Check sheet for the modelled part. Datum: model origin and axes. Units: mm. Face numbers are marked on the shaded views. Coordinates: 2 decimals unless noted, no trailing zeros. Loops run counter-clockwise (first coordinate to the right, second up) from the corner with the lowest first, then second, coordinate; pieces in that order, holes last. Notation, with made-up numbers: (-4, 63.5) - (38, 63.5) arc R17 ccw to (38, 77.5) - close; hole circle Ø8 at (83, 51). An arc over 180 degrees is marked (long way). Answer as a JSON object with one key per item and string values. Group by question number.
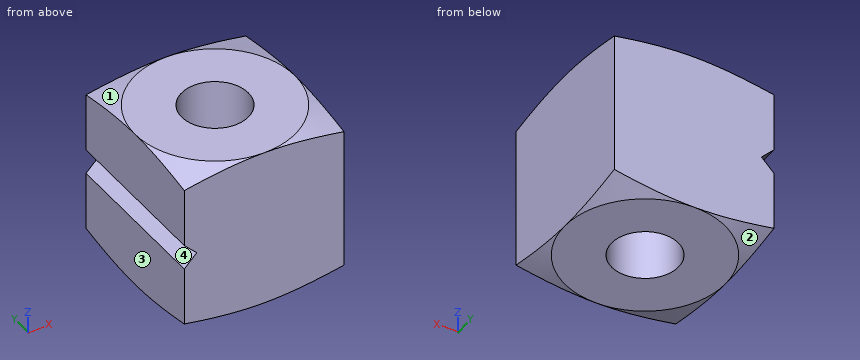
from build123d import *

# Parameters (mm, degrees)
F0_W      = 19.05
F0_H      = 19.05
F1_DEPTH  = 19.05
F2_R      = 3.96875
F3_DEPTH  = 19.051
F10_DEPTH = 12.7
F12_DEPTH = 25.4


with BuildPart() as f1:
    # F0 (on Top) → F1 (new body)
    with BuildSketch(Plane.XY):
        Rectangle(F0_W, F0_H)
    extrude(amount=F1_DEPTH)

    # F2 (on face) → F3 (cut, through all)
    with BuildSketch(Plane.XY.offset(19.05)):
        Circle(F2_R)
    extrude(amount=-F3_DEPTH, mode=Mode.SUBTRACT)

    # F4 (on Right) → F5 (revolve, cut)
    with BuildSketch(Plane.YZ):
        Polygon((24.765, 19.05), (9.525, 19.05), (24.765, 14.9664543073), align=None)
    revolve(axis=Axis((0, 0, 19.05), (0, 0, 1)), mode=Mode.SUBTRACT)

    # F7 (on Right) → F8 (revolve, cut)
    with BuildSketch(Plane.YZ):
        Polygon((-22.8305501432, 0), (-9.525, 0), (-22.8305501432, 3.5652114157), align=None)
    revolve(axis=Axis((0, 0, 0), (0, 0, -1)), mode=Mode.SUBTRACT)

    # F9 (on Front) → F10 (cut, symmetric)
    with BuildSketch(Plane.XZ):
        Polygon((-9.525, 8.7912914261), (-9.525, 9.525), (-10.3787914261, 7.9375), align=None)
    extrude(amount=F10_DEPTH, both=True, mode=Mode.SUBTRACT)

    # F11 (on face) → F12 (cut)
    with BuildSketch(Plane(origin=(0, 9.525, 0), x_dir=(-1, 0, 0), z_dir=(0, 1, 0))):
        Polygon((9.525, 8.0361114815), (9.525, 9.525), (8.0361114815, 9.525), align=None)
        Polygon((8.0361114815, 9.525), (9.525, 9.525), (9.525, 11.0138885185), align=None)
    extrude(amount=-F12_DEPTH, mode=Mode.SUBTRACT)


solid = f1.part
1. Gauge pin test, flat end, axial feed: pin 1 (5 mm diameter, centred on x = 0, y = -0.5, fed in from +Z). Record the tip position at first contact, or that the pin passes through.
2. Material ranges on line 1 (Y direction, x = 0, z = 6) (3 decimals); line 2 (Y direction, x = 1.75, z = 8) (3 decimals), recorded low to high.
3. Release check for a two-part mould opening along Z. For the marked faces 1, 2, 3 and 4 record: released by +Z, released by -Z, zero draft, split by the parting line, or undercut.
4. Sectioned sample at A-A on z = 4.5. Record the cut outline in (x, y) (1 decimal).
Answers follow:
{
 "1": {"pin 1": "passes through"},
 "2": {"line 1": "y = -9.525 to -3.969, 3.969 to 9.525", "line 2": "y = -9.525 to -3.562, 3.562 to 9.525"},
 "3": {"face 1": "released by +Z", "face 2": "released by -Z", "face 3": "zero draft", "face 4": "undercut"},
 "4": {"outline": "(-9.5, -9.5) - (9.5, -9.5) - (9.5, 9.5) - (-9.5, 9.5) - close; hole circle Ø7.9 at (0, 0)"}
}
